from build123d import *

# Parameters (mm, degrees)
SKETCH1_R               = 6
BOSS_EXTRUDE1_DEPTH     = 145
CHAMFER1_SIZE           = 0.5
CUT_EXTRUDE1_DEPTH      = 146.24806367
CUT_EXTRUDE1_DEPTH_BACK = 146.24806367
SKETCH2_W               = 1
SKETCH2_H               = 12


with BuildPart() as part:
    # Sketch1 → Boss-Extrude1 (new body)
    with BuildSketch(Plane(origin=(0, 0, 0), x_dir=(1, 0, 0), z_dir=(0, 1, 0))):
        with Locations(Location((0, 0, 0), (0, 0, 270))):
            Circle(SKETCH1_R)
    extrude(amount=BOSS_EXTRUDE1_DEPTH)

    # Chamfer1
    chamfer1_edges = [part.edges().sort_by_distance(p)[0] for p in [
        (0, 0, -6),
        (0, 145, -6),
    ]]
    chamfer(chamfer1_edges, length=CHAMFER1_SIZE)

    # Sketch2 → Cut-Extrude1 (cut, two sides: drawn at the far end of the back side and taken through both)
    with BuildSketch(Plane.XY.offset(-CUT_EXTRUDE1_DEPTH_BACK)):
        with Locations((5.5, 20)):
            Rectangle(SKETCH2_W, SKETCH2_H)
    extrude(amount=CUT_EXTRUDE1_DEPTH + CUT_EXTRUDE1_DEPTH_BACK, mode=Mode.SUBTRACT)


solid = part.part
Design review of the part built by this model. Coordinates are the model's own, in mm. A direction names the side the tool comes from. Give positions to 0.01 mm unless a question says otherwise; leave off trailing zeros. Order: outer loops, then holes, each group sorted by start corner. A loop starts at its lowest first (then second) coordinate and runs counter-clockwise, first axis right, second up.
1. For pin 1 Ø5 at (x, z) = (3, 4) entering from -Y; pin 2 Ø1 at (x, y) = (-4, 39) entering from -Z; pin 3 Ø2 at (x, y) = (-3.5, 71.5) entering from -Z; pin 4 Ø3 at (x, y) = (-2.5, 86) entering from +Z, all flat-tipped, find the tip position at first contact; note any pin that passes through.
Solution:
pin 1: stops at y = 0
pin 2: stops at z = -4.87
pin 3: stops at z = -5.45
pin 4: stops at z = 5.92
2. Add section B-B, the plane y = 96.5. State the section outline as (x, z) points.
Solution:
outline: circle Ø12 at (0, 0)
3. Tool access review of faces 1 (the flat face through (0, 145, 0)), 2 (the flat face through (5, 20, 0)): name each direction out of +Z, -Z, +X, -X, +Y, -Y from which nothing blocks a thin tool from reaching the whole face with its end or side.
Solution:
face 1: +Z, -Z, +X, -X, +Y
face 2: +Z, -Z, +X
4. To check wall thickness, follow L1, parallel to X at y = 77, z = 0.5; L2, parallel to Y at x = -4.25, z = -3.5. State the ranges of each line that lie inside material, in increasing order.
Solution:
L1: x = -5.98 to 5.98
L2: y = 0.01 to 144.99
5. Add section A-A, the plane y = 23.5. State the section outline as (x, z) points.
Solution:
outline: (5, -3.32) - (5, 3.32) arc R6 ccw (long way) to start
